Design review of the part built by this model. Coordinates are the model's own, in mm. A direction names the side the tool comes from. Round coordinates to 2 decimals unless told otherwise and drop trailing zeros. Order: outer loops, then holes, each group sorted by start corner. A loop starts at its lowest first (then second) coordinate and runs counter-clockwise, first axis right, second up. Notation, with made-up numbers: (9.25, 46) - (44.25, 46) arc R25 cw to (44.25, 80) - close; hole circle Ø10 at (50.25, 46). An arc over 180 degrees is marked (long way). Write item = value, one per line.
from build123d import *

# Parameters (mm, degrees)
SKETCH1_R           = 1.984375
SKETCH1_R_2         = 3.175
BOSS_EXTRUDE1_DEPTH = 3.175


with BuildPart() as part:
    # Sketch1 → Boss-Extrude1 (new body)
    with BuildSketch(Plane.XY):
        Polygon((25.4, 42.663065327), (25.4, -1.786934673), (50.8, -1.786934673), (50.8, 42.663065327), (101.6, 42.663065327), (101.6, 125.213065327), (25.4, 125.213065327), (25.4, 68.063065327), (0, 68.063065327), (0, 42.663065327), align=None)
        with Locations((38.1, 4.563065327)):
            Circle(SKETCH1_R, mode=Mode.SUBTRACT)
        with Locations((13.143553611, 55.363065327)):
            Circle(SKETCH1_R_2, mode=Mode.SUBTRACT)
        with Locations((38.1, 29.963065327)):
            Circle(SKETCH1_R, mode=Mode.SUBTRACT)
        with Locations((38.1, 55.363065327)):
            Circle(SKETCH1_R, mode=Mode.SUBTRACT)
        with Locations((63.5, 55.363065327)):
            Circle(SKETCH1_R, mode=Mode.SUBTRACT)
        with Locations((90.884375, 55.363065327)):
            Circle(SKETCH1_R, mode=Mode.SUBTRACT)
        with Locations((38.1, 80.763065327)):
            Circle(SKETCH1_R, mode=Mode.SUBTRACT)
        with Locations((38.1, 106.163065327)):
            Circle(SKETCH1_R, mode=Mode.SUBTRACT)
    extrude(amount=BOSS_EXTRUDE1_DEPTH)


solid = part.part
Item 1: Take a section at D-D, the plane y = 92. State the section outline as (x, z) points (3 decimals).
Data:
outline = (25.4, 0) - (101.6, 0) - (101.6, 3.175) - (25.4, 3.175) - close
Item 2: Insertion check: P1, Ø3.5, axis at x = 38.1, y = 4.56, coming from the +Z side; P2, Ø1, axis at x = 8, z = 2, coming from the -Y side; P3, Ø1, axis at y = 19.5, z = 1, coming from the -X side. Each pin has a flat end and moves straight along its axis. Give the tip position at first contact, or say it passes through.
Data:
P1 = through
P2 = 42.66
P3 = 25.4
Item 3: For faces 4 (the face through (13, 42.663, 2)), 5 (the face through (39.016, 53.603, 1.565)), 6 (the face through (76, 42.663, 2)), 7 (the face through (13, 68.063, 2)), list the 3-axis set-ups (+Z, -Z, +X, -X, +Y, -Y) from which the entire face can be reached by the end or side of a thin tool; tool diameter is ignored.
Data:
face_4 = +Z, -Z, -X, -Y
face_5 = +Z, -Z
face_6 = +Z, -Z, +X, -Y
face_7 = +Z, -Z, -X, +Y
Item 4: Take a section at A-A, the plane x = 38.1. State the section outline as (y, z) points (3 decimals).
Data:
outline = (-1.787, 0) - (2.579, 0) - (2.579, 3.175) - (-1.787, 3.175) - close; (6.547, 0) - (27.979, 0) - (27.979, 3.175) - (6.547, 3.175) - close; (31.947, 0) - (53.379, 0) - (53.379, 3.175) - (31.947, 3.175) - close; (57.347, 0) - (78.779, 0) - (78.779, 3.175) - (57.347, 3.175) - close; (82.747, 0) - (104.179, 0) - (104.179, 3.175) - (82.747, 3.175) - close; (108.147, 0) - (125.213, 0) - (125.213, 3.175) - (108.147, 3.175) - close
Item 5: Take a section at B-B, the plane x = 63.5. State the section outline as (y, z) points (3 decimals).
Data:
outline = (42.663, 0) - (53.379, 0) - (53.379, 3.175) - (42.663, 3.175) - close; (57.347, 0) - (125.213, 0) - (125.213, 3.175) - (57.347, 3.175) - close
Item 6: Take a section at C-C, the plane z = 2.3. Count the separate pieces of the cut face and the enclosed holes in it, and give its area (3 significant figures).
Data:
separate_pieces = 1
enclosed_holes = 8
area = 7,950 mm2
Item 7: For line 1 along Y through (x, z) = (38.1, 2.1); line 2 along Y through (x, z) = (63.5, 1.5); line 3 along X through (y, z) = (93.5, 2.65), list the stretches that pass through material, from the lowest coordinate up. Write a range as [from, to].
Data:
line_1 = [-1.79, 2.58], [6.55, 27.98], [31.95, 53.38], [57.35, 78.78], [82.75, 104.18], [108.15, 125.21]
line_2 = [42.66, 53.38], [57.35, 125.21]
line_3 = [25.4, 101.6]
Item 8: The part is to be moulded in two halves that separate along X. For faces 1 (the face through (0, 56, 2)), 2 (the face through (12.73, 58.51, 1.57)), 3 (the face through (50, 77, 3.175)), say which applies: +X half, -X half, draft (parallel to the pull), parting line (faces both ways), or undercut.
Data:
face_1 = -X half
face_2 = undercut
face_3 = draft
